Geometry check sheet. Reference: the model listing, model coordinates, mm. Face numbers are marked on the shaded views. A direction names the side the tool comes from. Round coordinates to 2 decimals unless told otherwise and drop trailing zeros. Order: outer loops, then holes, each group sorted by start corner. A loop starts at its lowest first (then second) coordinate and runs counter-clockwise, first axis right, second up. Notation, with made-up numbers: (33.25, 0.25) - (74.25, 0.25) arc R33 ccw to (74.25, 34.25) - close; hole circle Ø3 at (-11, -13.5). An arc over 180 degrees is marked (long way). Return JSON: item names as keys, results as strings. Group by question number.
Q1. Draft check along X on the marked faces 1, 2 and 3. Enter one of: pulls with the +X half, pulls with the -X half, needs draft (parallel to the pull), parting line crosses it, or undercut.
Q2. Material ranges on line 1 along Y through (x, z) = (0, -1.2); line 2 along Y through (x, z) = (0, -3.2); line 3 along Z through (x, y) = (2.5, 1), recorded low to high.
Q3. Sectioned sample at A-A, the plane x = 0. Record the cut outline in (y, z).
Q4. Tool access check on the marked faces 4 and 5. Record the directions out of +Z, -Z, +X, -X, +Y, -Y that give a thin tool (end or side, any length) a straight path to the whole face; none if there is none.
Q5. Sectioned sample at C-C, the plane z = -0.55. Record the cut outline in (x, y).
Q6. Gauge pin test, flat ends, axial feed: pin 1 Ø1.5 at (y, z) = (1.5, -0.5) entering from -X; pin 2 Ø1.5 at (y, z) = (3, -2.5) entering from -X. Record the tip position at first contact, or that the pin passes through.
```python
from build123d import *

# Parameters (mm, degrees)
F0_R     = 4
F1_DEPTH = 3
F2_R     = 2.5
F3_DEPTH = 1
F5_D     = 2.5
F6_SIZE  = 0.25


with BuildPart() as f1:
    # F0 (on Top) → F1 (new body)
    with BuildSketch(Plane.XY):
        Circle(F0_R)
    extrude(amount=-F1_DEPTH)

    # F2 (on face) → F3 (join)
    with BuildSketch(Plane(origin=(0, 0, -3), x_dir=(1, 0, 0), z_dir=(0, 0, -1))):
        Circle(F2_R)
    extrude(amount=F3_DEPTH)

    # F5 (through all)
    with Locations(Plane.XY):
        with Locations((0, 0)):
            Hole(F5_D / 2)

    # F6
    f6_edges = [f1.edges().sort_by_distance(p)[0] for p in [
        (-4, 0, 0),
        (-4, 0, -3),
        (-2.5, 0, -4),
        (-1.25, 0, 0),
    ]]
    chamfer(f6_edges, length=F6_SIZE)


solid = f1.part
```
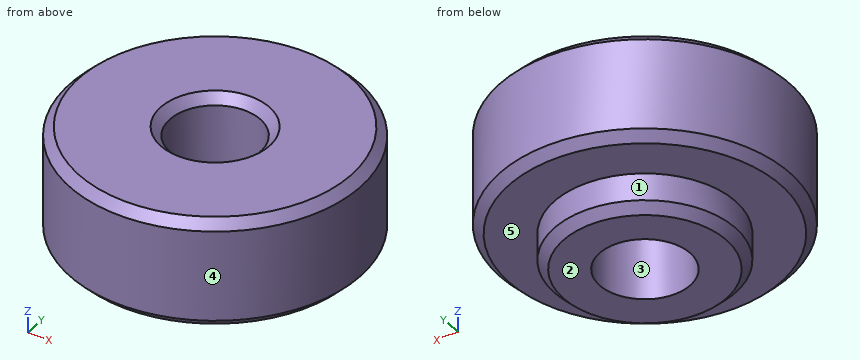
Reply:
{
 "1": {"face 1": "parting line crosses it", "face 2": "needs draft", "face 3": "undercut"},
 "2": {"line 1": "-4 to -1.25, 1.25 to 4", "line 2": "-2.5 to -1.25, 1.25 to 2.5", "line 3": "-3 to 0"},
 "3": {"outline": "(-4, -2.75) - (-3.75, -3) - (-2.5, -3) - (-2.5, -3.75) - (-2.25, -4) - (-1.25, -4) - (-1.25, -0.25) - (-1.5, 0) - (-3.75, 0) - (-4, -0.25) - close; (1.25, -4) - (2.25, -4) - (2.5, -3.75) - (2.5, -3) - (3.75, -3) - (4, -2.75) - (4, -0.25) - (3.75, 0) - (1.5, 0) - (1.25, -0.25) - close"},
 "4": {"face 4": "+Z, -Z", "face 5": "-Z"},
 "5": {"outline": "circle Ø8 at (0, 0); hole circle Ø2.5 at (0, 0)"},
 "6": {"pin 1": "x = -3.93", "pin 2": "x = -3.31"}
}
